Can you work these out from the drawing? Everything is in mm from the part's minimum corner. A direction names the side the tool comes from. Give positions to 0.01 mm unless a question says otherwise; leave off trailing zeros. Loops run counter-clockwise (first coordinate to the right, second up) from the corner with the lowest first, then second, coordinate; pieces in that order, holes last. Notation, with made-up numbers: (8, 15.5) -> (43, 15.5) arc R30 ccw to (43, 46.5) -> close; hole circle Ø2 at (77, 30.25). An arc over 180 degrees is marked (long way). Return JSON: item names as keys, results as strings. Group by question number.
Q1. Which directions (+Z, -Z, +X, -X, +Y, -Y) give clear straight access to the entire face, cutting with the end or side of a thin tool? Please do the marked faces 4 and 5.
Q2. Suppose I cut it at B-B, the plane z = 18.5. Please give me the cut outline in (x, y), and give its area (3 significant figures).
Q3. Suppose I cut it at D-D, the plane x = 38. Please give me the cut outline in (y, z), and give its area (3 significant figures).
Q4. Thinking about a two-plate mould opening in Y: for the marked faces 1, 2 and 3, which applies, pulls with the +Y half, pulls with the -Y half, needs draft (parallel to the pull), parting line crosses it, or undercut?
Q5. I need wall thicknesses on line 1 along X through (y, z) = (39.1, 12.5); line 2 along Y through (x, z) = (41, 4.5); line 3 along Z through (x, y) = (49.5, 39.2). Which ranges of each line are inside material? Lowest first, please. Write a range as [from, to].
Q6. Will these pins go through, and if not, where does the flat tip stop? pin 1 (2.5 mm diameter, centred on x = 49.5, z = 12.5, fed in from -Y); pin 2 (12 mm diameter, centred on x = 21, y = 19.5, fed in from -Z); pin 3 (1.6 mm diameter, centred on y = 0.5, z = 26, fed in from +X); pin 4 (5 mm diameter, centred on x = 49.5, z = 12.5, fed in from -Y).
Q7. Suppose I cut it at A-A, the plane z = 12.5. Please give me the cut outline in (x, y), and give its area (3 significant figures).
Q8. Suppose I cut it at C-C, the plane x = 20.5. Please give me the cut outline in (y, z), and give its area (3 significant figures).
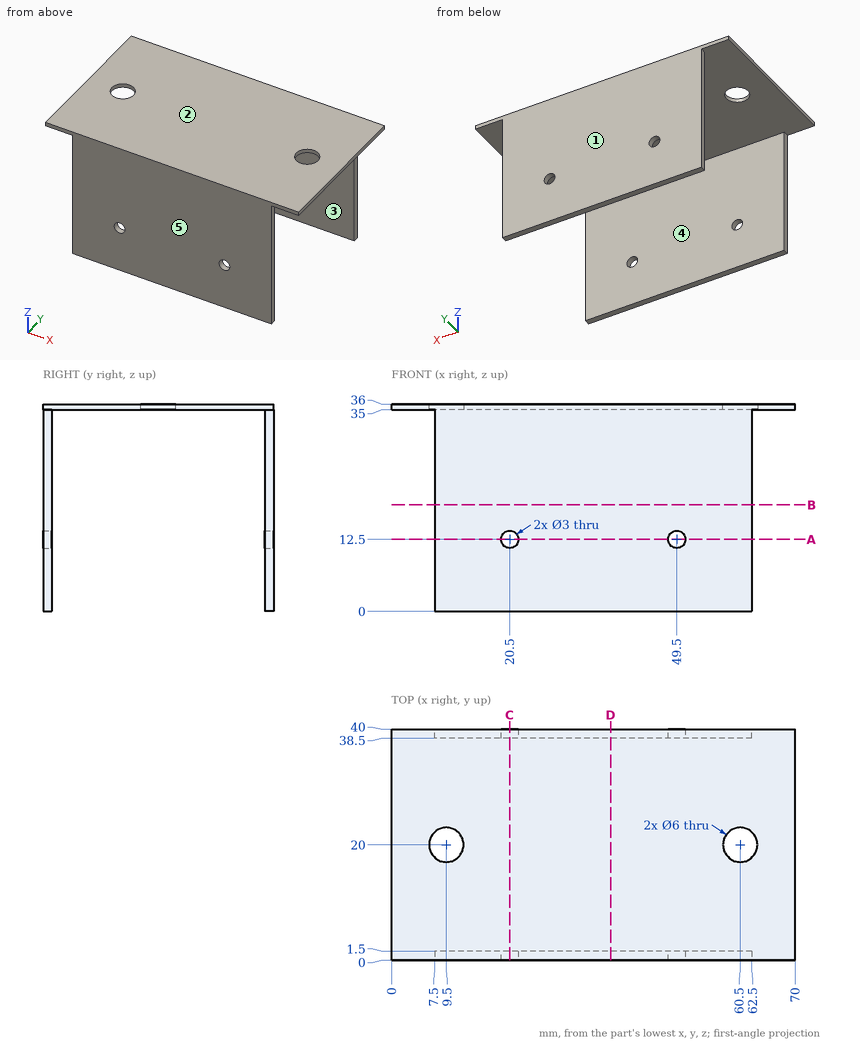
Ans:
{
 "1": {"face 4": "-Z, +X, -X", "face 5": "+Z, -Z, +X, -X, -Y"},
 "2": {"outline": "(7.5, 0) -> (62.5, 0) -> (62.5, 1.5) -> (7.5, 1.5) -> close; (7.5, 38.5) -> (62.5, 38.5) -> (62.5, 40) -> (7.5, 40) -> close", "area": "165 mm^2"},
 "3": {"outline": "(0, 0) -> (1.5, 0) -> (1.5, 35) -> (38.5, 35) -> (38.5, 0) -> (40, 0) -> (40, 36) -> (0, 36) -> close", "area": "145 mm^2"},
 "4": {"face 1": "pulls with the +Y half", "face 2": "needs draft", "face 3": "undercut"},
 "5": {"line 1": "x = [7.5, 19], [22, 48], [51, 62.5]", "line 2": "y = [0, 1.5], [38.5, 40]", "line 3": "z = [0, 11], [14, 36]"},
 "6": {"pin 1": "passes through", "pin 2": "stops at z = 35", "pin 3": "stops at x = 62.5", "pin 4": "stops at y = 0"},
 "7": {"outline": "(7.5, 0) -> (19, 0) -> (19, 1.5) -> (7.5, 1.5) -> close; (7.5, 38.5) -> (19, 38.5) -> (19, 40) -> (7.5, 40) -> close; (22, 0) -> (48, 0) -> (48, 1.5) -> (22, 1.5) -> close; (22, 38.5) -> (48, 38.5) -> (48, 40) -> (22, 40) -> close; (51, 0) -> (62.5, 0) -> (62.5, 1.5) -> (51, 1.5) -> close; (51, 38.5) -> (62.5, 38.5) -> (62.5, 40) -> (51, 40) -> close", "area": "147 mm^2"},
 "8": {"outline": "(0, 0) -> (1.5, 0) -> (1.5, 11) -> (0, 11) -> close; (0, 14) -> (1.5, 14) -> (1.5, 35) -> (38.5, 35) -> (38.5, 14) -> (40, 14) -> (40, 36) -> (0, 36) -> close; (38.5, 0) -> (40, 0) -> (40, 11) -> (38.5, 11) -> close", "area": "136 mm^2"}
}
